from build123d import *

# Parameters (mm, degrees)
SKETCH2_W           = 220
SKETCH2_H           = 220
BOSS_EXTRUDE2_DEPTH = 10
SKETCH3_R           = 1.5
CUT_EXTRUDE2_DEPTH  = 10
SKETCH4_R           = 1.5
SKETCH4_W           = 10
SKETCH4_H           = 24
CUT_EXTRUDE3_DEPTH  = 10
SKETCH6_R           = 2
CUT_EXTRUDE4_DEPTH  = 10


with BuildPart() as part:
    # Sketch2 → Boss-Extrude2 (new body)
    with BuildSketch(Plane.XY):
        with Locations((222.522330277, 20.812483699)):
            Rectangle(SKETCH2_W, SKETCH2_H)
    extrude(amount=BOSS_EXTRUDE2_DEPTH)

    # Sketch3 → Cut-Extrude2 (cut)
    with BuildSketch(Plane.XY.offset(10)):
        with Locations((117.522330277, 125.812483699)):
            Circle(SKETCH3_R)
        with Locations((117.522330277, -84.187516301)):
            Circle(SKETCH3_R)
        with Locations((327.522330277, -84.187516301)):
            Circle(SKETCH3_R)
        with Locations((327.522330277, 125.812483699)):
            Circle(SKETCH3_R)
    extrude(amount=-CUT_EXTRUDE2_DEPTH, mode=Mode.SUBTRACT)

    # Sketch4 → Cut-Extrude3 (cut)
    with BuildSketch(Plane.XY.offset(10)):
        with Locations((128.522330277, 58.812483699)):
            Circle(SKETCH4_R)
        with Locations((148.522330277, 58.812483699)):
            Circle(SKETCH4_R)
        with Locations((128.522330277, 12.812483699)):
            Circle(SKETCH4_R)
        with Locations((148.522330277, 12.812483699)):
            Circle(SKETCH4_R)
        with Locations((296.522330277, 12.812483699)):
            Circle(SKETCH4_R)
        with Locations((316.522330277, 12.812483699)):
            Circle(SKETCH4_R)
        with Locations((296.522330277, 58.812483699)):
            Circle(SKETCH4_R)
        with Locations((316.522330277, 58.812483699)):
            Circle(SKETCH4_R)
        with Locations((138.522330277, 58.812483699)):
            Rectangle(SKETCH4_W, SKETCH4_H)
        with Locations((138.522330277, 12.812483699)):
            Rectangle(SKETCH4_W, SKETCH4_H)
        with Locations((306.522330277, 58.812483699)):
            Rectangle(SKETCH4_W, SKETCH4_H)
        with Locations((306.522330277, 12.812483699)):
            Rectangle(SKETCH4_W, SKETCH4_H)
    extrude(amount=-CUT_EXTRUDE3_DEPTH, mode=Mode.SUBTRACT)

    # Sketch6 → Cut-Extrude4 (cut)
    with BuildSketch(Plane.XY.offset(10)):
        with Locations((222.522330277, 39.812483699)):
            Circle(SKETCH6_R)
        with Locations((222.522330277, 1.812483699)):
            Circle(SKETCH6_R)
    extrude(amount=-CUT_EXTRUDE4_DEPTH, mode=Mode.SUBTRACT)


solid = part.part
For this review, take the finished solid that the model builds, in its own axes (mm). A direction names the side the tool comes from. Round coordinates to 2 decimals unless told otherwise and drop trailing zeros. Write each loop counter-clockwise with the first axis right and the second up, starting at its lowest first coordinate (ties: lowest second). Pieces come first, ordered by that corner, then holes. Notation, with made-up numbers: (82, 58.25) - (114, 58.25) arc R7 cw to (114, 71.25) - close; hole circle Ø7 at (-16.5, -32). An arc over 180 degrees is marked (long way). Write item = value, one per line. Start each with the question number.
1. Draft analysis for pull direction Y (two halves, no side actions). For faces 1 (the face through (221, 130.812, 5)), 2 (the face through (332.522, 19, 5)), 3 (the face through (306, 0.812, 5)), state which applies: released by +Y, released by -Y, zero draft, split by the parting line, or undercut.
2. For faces 4 (the face through (221, -89.188, 5)), 5 (the face through (138, 70.812, 5)), list the 3-axis set-ups (+Z, -Z, +X, -X, +Y, -Y) from which the entire face can be reached by the end or side of a thin tool; tool diameter is ignored.
3. Consider section B-B on z = 1.75. Give the number of separate pieces and of enclosed holes in the cut face, plus the area to 3 significant figures.
4. Consider section A-A on y = 63.5. State the section outline as (x, z) points.
5. Wall thickness on L1, parallel to Y at x = 304, z = 3.5; L2, parallel to X at y = 4, z = 4; L3, parallel to X at y = 2.5, z = 3: over which ranges is each line inside the solid? List them lowest first.
Evaluation:
q1.face_1 = released by +Y
q1.face_2 = zero draft
q1.face_3 = undercut
q2.face_4 = +Z, -Z, +X, -X, -Y
q2.face_5 = +Z, -Z
q3.separate_pieces = 1
q3.enclosed_holes = 18
q3.area = 47,300 mm2
q4.outline = (112.52, 0) - (133.52, 0) - (133.52, 10) - (112.52, 10) - close; (143.52, 0) - (301.52, 0) - (301.52, 10) - (143.52, 10) - close; (311.52, 0) - (332.52, 0) - (332.52, 10) - (311.52, 10) - close
q5.L1 = -89.19 to 0.81, 24.81 to 46.81, 70.81 to 130.81
q5.L2 = 112.52 to 133.52, 143.52 to 301.52, 311.52 to 332.52
q5.L3 = 112.52 to 133.52, 143.52 to 220.64, 224.4 to 301.52, 311.52 to 332.52
